```python
from build123d import *

# Parameters (mm, degrees)
SKETCH1_W                = 54.25
SKETCH1_H                = 165
BOSS_EXTRUDE1_DEPTH      = 9.6
BOSS_EXTRUDE2_DEPTH      = 1.55
BOSS_EXTRUDE2_DEPTH_BACK = 1.55
SKETCH2_W                = 4.25
SKETCH2_H                = 4.9
SKETCH15_W               = 4.25
SKETCH15_H               = 4.9
CUT_EXTRUDE1_DEPTH       = 1.55
SKETCH17_W               = 2
SKETCH17_H               = 165
CUT_EXTRUDE2_DEPTH       = 2.7


with BuildPart() as part:
    # Sketch1 → Boss-Extrude1 (new body)
    with BuildSketch(Plane(origin=(0, 0, 0), x_dir=(1, 0, 0), z_dir=(0, 1, 0))):
        Rectangle(SKETCH1_W, SKETCH1_H)
    extrude(amount=-BOSS_EXTRUDE1_DEPTH)

    # Sketch2 → Boss-Extrude2 (add, two sides: drawn at the far end of the back side and taken through both)
    with BuildSketch(Plane(origin=(27.125, 0, 0), x_dir=(0, 0, -1), z_dir=(1, 0, 0)).offset(-BOSS_EXTRUDE2_DEPTH_BACK)):
        with Locations((-67.575, -7.15)):
            Rectangle(SKETCH2_W, SKETCH2_H)
        with Locations((67.575, -7.15)):
            Rectangle(SKETCH2_W, SKETCH2_H)
        with Locations((0, -7.15)):
            Rectangle(SKETCH2_W, SKETCH2_H)
    extrude(amount=BOSS_EXTRUDE2_DEPTH + BOSS_EXTRUDE2_DEPTH_BACK)

    # Sketch15 → Cut-Extrude1 (cut)
    with BuildSketch(Plane.ZY.offset(27.125)):
        with Locations((67.575, -7.15)):
            Rectangle(SKETCH15_W, SKETCH15_H)
        with Locations((-67.575, -7.15)):
            Rectangle(SKETCH15_W, SKETCH15_H)
        with Locations((0, -7.15)):
            Rectangle(SKETCH15_W, SKETCH15_H)
    extrude(amount=-CUT_EXTRUDE1_DEPTH, mode=Mode.SUBTRACT)

    # Sketch17 → Cut-Extrude2 (cut)
    with BuildSketch(Plane(origin=(0, 0, 0), x_dir=(1, 0, 0), z_dir=(0, 1, 0))):
        Rectangle(SKETCH17_W, SKETCH17_H)
    extrude(amount=-CUT_EXTRUDE2_DEPTH, mode=Mode.SUBTRACT)


solid = part.part
```
Part model, mm, in its own coordinate system. A direction names the side the tool comes from. Round coordinates to 2 decimals unless told otherwise and drop trailing zeros. Loops run counter-clockwise (first coordinate to the right, second up) from the corner with the lowest first, then second, coordinate; pieces in that order, holes last. Notation, with made-up numbers: (-30, 17) -> (25, 17) arc R30 ccw to (25, 46) -> close; hole circle Ø7 at (53.25, 87.25). An arc over 180 degrees is marked (long way). Use CSV: the item, a comma, the result in double quotes. Start each with the question number.
1) Wall check: L1, parallel to X at y = -2, z = 17 (3 decimals); L2, parallel to X at y = -7.5, z = 11 (3 decimals); L3, parallel to Y at x = 0, z = 22.5. Give the ranges that are in metal, low to high. Write a range as [from, to].
2) Drop flat-ended pins along their axis: P1, Ø1.2, axis at x = 28, z = -67, coming from the +Y side; P2, Ø0.8, axis at x = -26.5, z = 68.5, coming from the -Y side; P3, Ø0.8, axis at x = 28, y = -7, coming from the -Z side. Give the stop position or say it passes through.
3) Pull direction Z, two halves, no side cores. Call faces 4 (the flat face through (28.675, -7, -68)), 5 (the flat face through (-25.575, -7, -68)), 6 (the flat face through (0, -5, -82.5)), 7 (the flat face through (-25.575, -7, 0)): +Z half, -Z half, draft (parallel to the pull), parting line (faces both ways), or undercut.
4) Which spindle directions (+Z, -Z, +X, -X, +Y, -Y) get a long thin tool onto all of the face, cutting with end or side? Do faces 1 (the flat face through (1, -1, 1)), 2 (the flat face through (-25.575, -7, 68)), 3 (the flat face through (0, -5, 82.5)). Say none if no direction does.
5) Cut at A-A, the plane z = -0.5. Write the cut outline in (x, y) (3 decimals).
6) Cut at B-B, the plane y = -7.5. Write the cut outline in (x, z) (3 decimals).
Determined:
1,L1,"x = [-27.125, -1], [1, 27.125]"
1,L2,"x = [-27.125, 27.125]"
1,L3,"y = [-9.6, -2.7]"
2,P1,"stops at y = -4.7"
2,P2,"stops at y = -4.7"
2,P3,"stops at z = -69.7"
3,face 4,"draft"
3,face 5,"undercut"
3,face 6,"-Z half"
3,face 7,"undercut"
4,face 1,"+Z, -Z, +Y"
4,face 2,"-X, -Y"
4,face 3,"+Z, +X, -X, +Y, -Y"
5,outline,"(-27.125, -4.7) -> (-25.575, -4.7) -> (-25.575, -9.6) -> (28.675, -9.6) -> (28.675, -4.7) -> (27.125, -4.7) -> (27.125, 0) -> (1, 0) -> (1, -2.7) -> (-1, -2.7) -> (-1, 0) -> (-27.125, 0) -> close"
6,outline,"(-27.125, -82.5) -> (27.125, -82.5) -> (27.125, -69.7) -> (28.675, -69.7) -> (28.675, -65.45) -> (27.125, -65.45) -> (27.125, -2.125) -> (28.675, -2.125) -> (28.675, 2.125) -> (27.125, 2.125) -> (27.125, 65.45) -> (28.675, 65.45) -> (28.675, 69.7) -> (27.125, 69.7) -> (27.125, 82.5) -> (-27.125, 82.5) -> (-27.125, 69.7) -> (-25.575, 69.7) -> (-25.575, 65.45) -> (-27.125, 65.45) -> (-27.125, 2.125) -> (-25.575, 2.125) -> (-25.575, -2.125) -> (-27.125, -2.125) -> (-27.125, -65.45) -> (-25.575, -65.45) -> (-25.575, -69.7) -> (-27.125, -69.7) -> close"
